Check sheet for the drawn part. Datum: minimum x, y, z corner. Units: mm. Give positions to 0.01 mm unless a question says otherwise; leave off trailing zeros. Order: outer loops, then holes, each group sorted by start corner. A loop starts at its lowest first (then second) coordinate and runs counter-clockwise, first axis right, second up. Notation, with made-up numbers: (18, 78) -> (42, 78) arc R18 ccw to (42, 108) -> close; hole circle Ø10 at (62, 14.25). An arc over 180 degrees is marked (long way). Answer in a Markdown table with one row per item. Add a question column.
(1) Go/stop test with flat-tipped pins: pin 1 (2.5 mm diameter, centred on x = 8.5, z = 124.5, fed in from -Y) (1 decimal); pin 2 (5.5 mm diameter, centred on y = 115.75, z = 40.75, fed in from -X); pin 3 (1.7 mm diameter, centred on x = 11.5, z = 2, fed in from +Y) (1 decimal). Record where each tip stops, or that it passes through.
(2) Cross-section at B-B (y = 52.5). Record the cut outline in (x, z) (1 decimal), then the cut area to 3 significant figures.
(3) Thickness scan on L1, parallel to X at y = 13, z = 98.5; L2, parallel to Y at x = 12, z = 116.5 (1 decimal); L3, parallel to Z at x = 25, y = 17 (1 decimal). Record the ranges inside material, lowest first. Write a range as [from, to].
(4) Release check for a two-part mould opening along Z. For the marked faces 1, 2 and 3 record: released by +Z, released by -Z, zero draft, split by the parting line, or undercut.
(5) Cross-section at D-D (y = 18.5). Record the cut outline in (x, z).
(6) Cross-section at A-A (x = 24). Record the cut outline in (y, z) (1 decimal).
(7) Cross-section at C-C (z = 89). Record the cut outline in (x, y) (1 decimal).
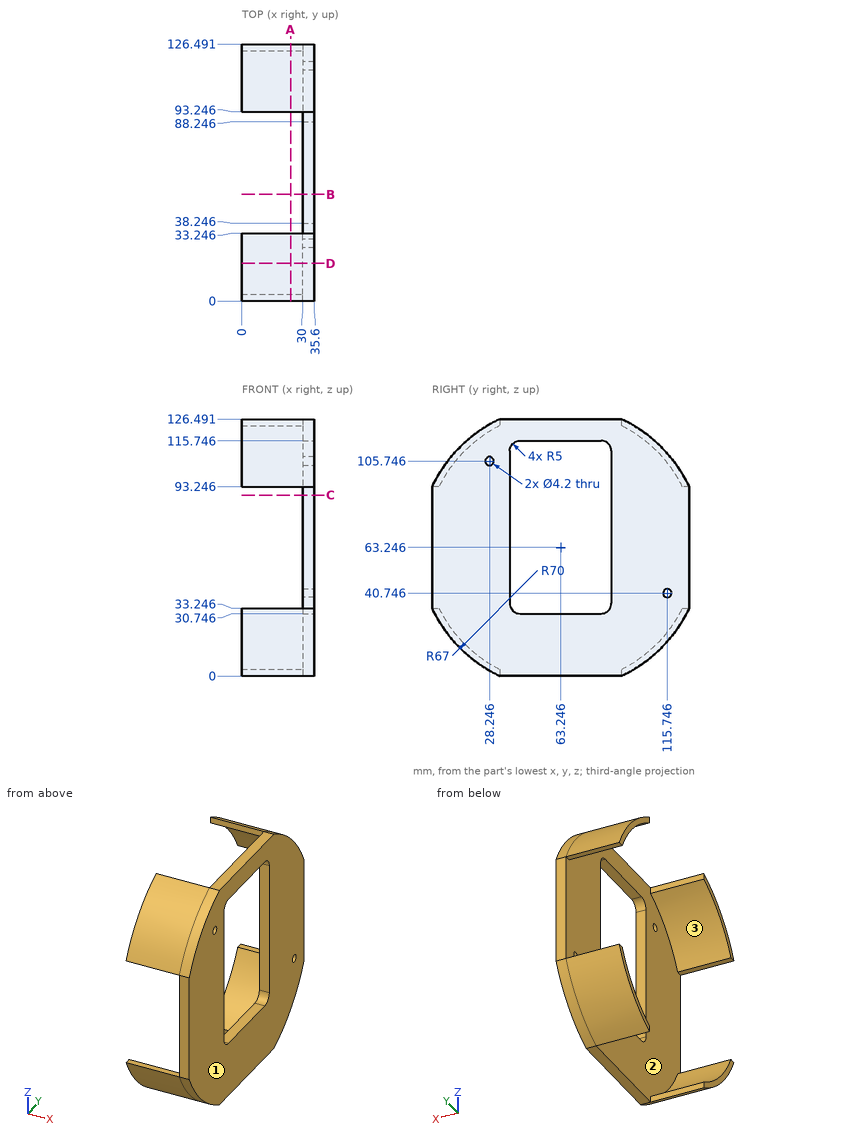
Answer below:
| question | item | result |
|---|---|---|
| 1 | pin 1 | stops at y = 27.2 |
| 1 | pin 2 | stops at x = 30 |
| 1 | pin 3 | stops at y = 98.6 |
| 2 | outline | (30, 0) -> (35.6, 0) -> (35.6, 30.7) -> (30, 30.7) -> close; (30, 115.7) -> (35.6, 115.7) -> (35.6, 126.5) -> (30, 126.5) -> close |
| 2 | area | 232 mm² |
| 3 | L1 | x = [30, 35.6] |
| 3 | L2 | y = [17.8, 22.6], [103.9, 108.7] |
| 3 | L3 | z = [10.7, 14.8], [111.7, 115.8] |
| 4 | face 1 | zero draft |
| 4 | face 2 | undercut |
| 4 | face 3 | undercut |
| 5 | outline | (0, 9.41) -> (35.6, 9.41) -> (35.6, 117.08) -> (0, 117.08) -> (0, 113.11) -> (30, 113.11) -> (30, 13.38) -> (0, 13.38) -> close |
| 6 | outline | (0, 33.2) arc R70 ccw to (33.2, 0) -> (33.2, 3.3) arc R67 cw to (3.3, 33.2) -> close; (0, 93.2) -> (3.3, 93.2) arc R67 cw to (33.2, 123.2) -> (33.2, 126.5) arc R70 ccw to start; (93.2, 0) arc R70 ccw to (126.5, 33.2) -> (123.2, 33.2) arc R67 cw to (93.2, 3.3) -> close; (93.2, 123.2) arc R67 cw to (123.2, 93.2) -> (126.5, 93.2) arc R70 ccw to (93.2, 126.5) -> close |
| 7 | outline | (30, 0) -> (35.6, 0) -> (35.6, 38.2) -> (30, 38.2) -> close; (30, 88.2) -> (35.6, 88.2) -> (35.6, 126.5) -> (30, 126.5) -> close |
